Work out the finished part from the listing and answer in its coordinate system (mm). A direction names the side the tool comes from. Give positions to 0.01 mm unless a question says otherwise; leave off trailing zeros. Write each loop counter-clockwise with the first axis right and the second up, starting at its lowest first coordinate (ties: lowest second). Pieces come first, ordered by that corner, then holes.
1) Find section D-D (z = 11.75). Determine the outline of the cut face in (x, y).
2) Find section A-A (y = -3.75). Determine the outline of the cut face in (x, z).
3) Straight lines are drawn through the part: probe 1 along Y at (x, z) = (0, 5.75); probe 2 along Z at (x, y) = (2.75, -2); probe 3 along Y at (x, z) = (0, 3.95). For each, find the intervals that lie inside material, in ascending order.
4) Determine the mould class of faces 1 (the face through (-0.59, 4.46, 10.94)), 2 (the face through (0, 0, 17)), 3 (the face through (-5.158, -3.955, 8.381)) for opening direction X: pulls with the +X half, pulls with the -X half, needs draft (parallel to the pull), parting line crosses it, or undercut.
5) A tool of negligible diameter and unlimited length cuts with its end or side. For faces 4 (the face through (-0.59, 4.46, 2.46)), 5 (the face through (0, 0, 15)), 6 (the face through (-4.42, 1.54, 0)), from which of +Z, -Z, +X, -X, +Y, -Y can it reach the whole face along a straight path? Write none if from no direction.
6) Given pin 1 Ø2 at (y, z) = (2, 12) entering from +X; pin 2 Ø1 at (x, z) = (3, 3) entering from -Y; pin 3 Ø4.5 at (x, y) = (0, -0.5) entering from -Z, each flat-ended and moving along its own axis, determine where each tip first touches the part or whether it passes through.
7) Find section B-B (x = 0). Determine the outline of the cut face in (y, z), plus the area to 3 significant figures.
```python
from build123d import *

# Parameters (mm, degrees)
F0_R     = 6.5
F0_R_2   = 4.5
F1_DEPTH = 17
F2_START = 5
F0_R_3   = 3
F2_DEPTH = 2
F3_START = 15
F3_DEPTH = 2


with BuildPart() as f1:
    # F0 (on Top) → F1 (new body)
    with BuildSketch(Plane.XY):
        Circle(F0_R)
        Circle(F0_R_2, mode=Mode.SUBTRACT)
    extrude(amount=F1_DEPTH)

    # F0 (on Top) → F2 (join)
    with BuildSketch(Plane.XY.offset(F2_START)):
        Circle(F0_R_2)
        Circle(F0_R_3, mode=Mode.SUBTRACT)
    extrude(amount=F2_DEPTH)

    # F0 (on Top) → F3 (join)
    with BuildSketch(Plane.XY.offset(F3_START)):
        Circle(F0_R_2)
        Circle(F0_R_3, mode=Mode.SUBTRACT)
        Circle(F0_R_3)
    extrude(amount=F3_DEPTH)


solid = f1.part
```
Results:
1. outline: circle Ø13 at (0, 0); hole circle Ø9 at (0, 0)
2. outline: (-5.31, 0) - (-2.49, 0) - (-2.49, 5) - (2.49, 5) - (2.49, 0) - (5.31, 0) - (5.31, 17) - (-5.31, 17) - close; hole (-2.49, 7) - (2.49, 7) - (2.49, 15) - (-2.49, 15) - close
3. probe 1: y = -6.5 to -3, 3 to 6.5
3. probe 2: z = 5 to 7, 15 to 17
3. probe 3: y = -6.5 to -4.5, 4.5 to 6.5
4. face 1: undercut
4. face 2: needs draft
4. face 3: parting line crosses it
5. face 4: -Z
5. face 5: none
5. face 6: -Z, +X, -X, +Y, -Y
6. pin 1: stops at x = 6.42
6. pin 2: stops at y = -6
6. pin 3: stops at z = 15
7. outline: (-6.5, 0) - (-4.5, 0) - (-4.5, 5) - (-3, 5) - (-3, 7) - (-4.5, 7) - (-4.5, 15) - (4.5, 15) - (4.5, 7) - (3, 7) - (3, 5) - (4.5, 5) - (4.5, 0) - (6.5, 0) - (6.5, 17) - (-6.5, 17) - close
7. area: 92.0 mm2
